```python
from build123d import *

# Parameters (mm, degrees)
F0_W     = 1450
F0_H     = 2400
F1_DEPTH = 500
F2_T     = -18
F4_DEPTH = 482
F5_W     = 1414.227886
F5_H     = 18
F5_W_2   = 482
F6_DEPTH = 482


with BuildPart() as f1:
    # F0 (on Front) → F1 (new body)
    with BuildSketch(Plane.XZ):
        Rectangle(F0_W, F0_H)
    extrude(amount=F1_DEPTH)

    # F2
    f2_openings = [f1.faces().sort_by_distance(p)[0] for p in [
        (0, -500, 0),
    ]]
    offset(amount=F2_T, openings=f2_openings)

    # F3 (on face) → F4 (join)
    with BuildSketch(Plane.XZ.offset(18)):
        Polygon((707, 800), (-707, 800), (-707, 782), (-225, 782), (-225, -700), (-707, -700), (-707, -718), (-9, -718), (-9, -941), (-707, -941), (-707, -959), (-9, -959), (-9, -1182), (9, -1182), (9, -959), (707, -959), (707, -941), (9, -941), (9, -718), (707, -718), (707, -700), (-207, -700), (-207, 782), (707, 782), align=None)
    extrude(amount=F4_DEPTH)

    # F5 (on face) → F6 (join)
    with BuildSketch(Plane.XZ.offset(18)):
        with Locations((0.113943, -359)):
            Rectangle(F5_W, F5_H)
        with Locations((-466, -18)):
            Rectangle(F5_W_2, F5_H)
    extrude(amount=F6_DEPTH)


solid = f1.part
```
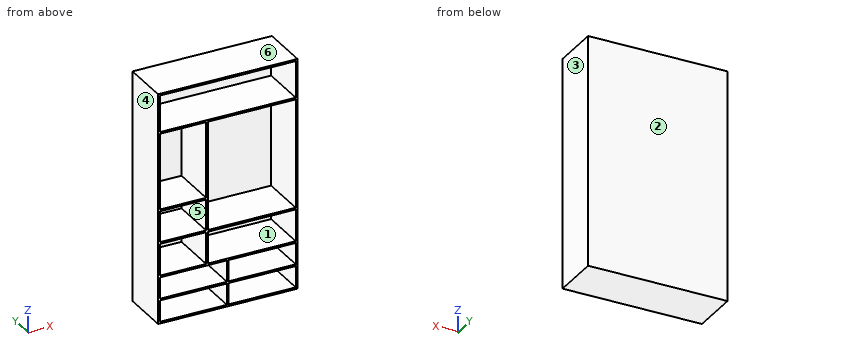
Input: part model. Units: mm. Frame: model coordinates. Face numbers are marked on the shaded views. A direction names the side the tool comes from. Give positions to 0.01 mm unless a question says otherwise; leave off trailing zeros. Order: outer loops, then holes, each group sorted by start corner. A loop starts at its lowest first (then second) coordinate and runs counter-clockwise, first axis right, second up. Notation, with made-up numbers: (87, 2.5) - (139, 2.5) arc R16 ccw to (139, 22.5) - close; hole circle Ø5 at (42.5, 87.25). An arc over 180 degrees is marked (long way). Use a Markdown table: item, result.
(1) Section query D-D (x = 42). Output: boundary loops of the cut face in (y, z).
Computed values:
| item | result |
|---|---|
| outline | (-500, -1200) - (0, -1200) - (0, 1200) - (-500, 1200) - (-500, 1182) - (-18, 1182) - (-18, 800) - (-500, 800) - (-500, 782) - (-18, 782) - (-18, -350) - (-500, -350) - (-500, -368) - (-18, -368) - (-18, -700) - (-500, -700) - (-500, -718) - (-18, -718) - (-18, -941) - (-500, -941) - (-500, -959) - (-18, -959) - (-18, -1182) - (-500, -1182) - close |
(2) Draft query along X for the marked faces 3, 4, 5 and 6. Return one class per face: released by +X, released by -X, zero draft, split by the parting line, or undercut.
Computed values:
| item | result |
|---|---|
| face 3 | released by +X |
| face 4 | released by -X |
| face 5 | undercut |
| face 6 | zero draft |
(3) Section query B-B (z = 908.5). Output: boundary loops of the cut face in (x, y), then the cut area to 3 significant figures.
Computed values:
| item | result |
|---|---|
| outline | (-725, -500) - (-707, -500) - (-707, -18) - (707, -18) - (707, -500) - (725, -500) - (725, 0) - (-725, 0) - close |
| area | 43,500 mm2 |
(4) Section query C-C (y = -420.5). State how many separate pieces and enclosed holes the cut face has, then the cut area to 3 significant figures.
Computed values:
| item | result |
|---|---|
| separate pieces | 1 |
| enclosed holes | 10 |
| area | 282,000 mm2 |
(5) Section query A-A (x = -478). Output: boundary loops of the cut face in (y, z).
Computed values:
| item | result |
|---|---|
| outline | (-500, -1200) - (0, -1200) - (0, 1200) - (-500, 1200) - (-500, 1182) - (-18, 1182) - (-18, 800) - (-500, 800) - (-500, 782) - (-18, 782) - (-18, -9) - (-500, -9) - (-500, -27) - (-18, -27) - (-18, -350) - (-500, -350) - (-500, -368) - (-18, -368) - (-18, -700) - (-500, -700) - (-500, -718) - (-18, -718) - (-18, -941) - (-500, -941) - (-500, -959) - (-18, -959) - (-18, -1182) - (-500, -1182) - close |
(6) Pin query (flat end, axial travel): pin 1 (6 mm diameter, centred on x = -170.5, z = 606, fed in from -Y). Return the tip coordinate at first contact, or that it passes through.
Computed values:
| item | result |
|---|---|
| pin 1 | stops at y = -18 |
(7) Line query: line 1 (Z direction, x = -154.5, y = -277); line 2 (X direction, y = -123, z = -1006); line 3 (X direction, y = -55, z = 612.5). Output: solid intervals per line, ascending. Write a range as from..to.
Computed values:
| item | result |
|---|---|
| line 1 | z = -1200..-1182, -959..-941, -718..-700, -368..-350, 782..800, 1182..1200 |
| line 2 | x = -725..-707, -9..9, 707..725 |
| line 3 | x = -725..-707, -225..-207, 707..725 |
(8) Access query for the marked faces 1 and 2. Directions: +Z, -Z, +X, -X, +Y, -Y. A direction counts if a zero-diameter tool reaches every point of the face in a straight line with its end or side. Return the directions, or none.
Computed values:
| item | result |
|---|---|
| face 1 | -Y |
| face 2 | +Z, -Z, +X, -X, +Y |
